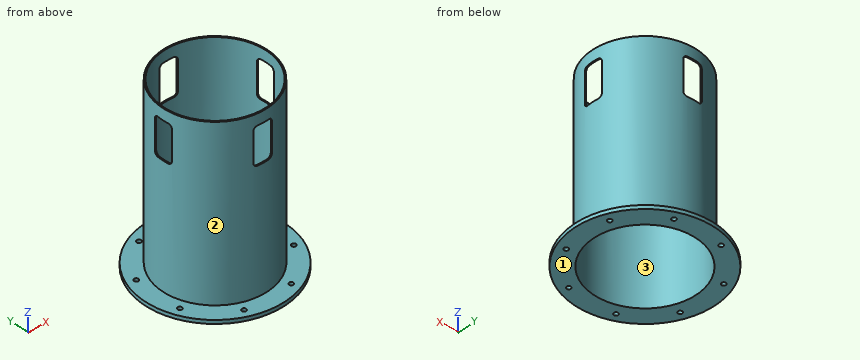
from build123d import *

# Parameters (mm, degrees)
SKETCH011_R      = 17.5
EXTRUDE005_DEPTH = 30
ARRAY004_COUNT   = 8
EXTRUDE_DEPTH    = 500
ARRAY_COUNT      = 4


with BuildPart() as extrude005:
    # Sketch011 (on Face4 of Cut) → Extrude005 (new body)
    with BuildSketch(Plane(origin=(0, 0, 2955), x_dir=(1, 0, 0), z_dir=(0, 0, -1))):
        with Locations((461.939766, 191.341716)):
            Circle(SKETCH011_R)
    extrude(amount=-EXTRUDE005_DEPTH)


with BuildPart() as array004:
    # Array004 base: copy of Extrude005
    add(extrude005.part)

    # Array004: Array004 ×8 about axis
    array004_axis = Axis((0, 0, 0), (0, 0, 1))


with BuildPart() as array004_1:
    add(array004.part)
    for i in range(1, ARRAY004_COUNT):
        add(array004.part.rotate(array004_axis, i * 360 / ARRAY004_COUNT))


with BuildPart() as array:
    # Sketch010 → Extrude (new body)
    with BuildSketch(Plane.XZ):
        with BuildLine():
            Line((-45, 3965), (45, 3965))
            ThreePointArc((45, 3965), (66.213203, 3973.786797), (75, 3995))
            Line((75, 3995), (75, 4235))
            ThreePointArc((75, 4235), (66.213203, 4256.213203), (45, 4265))
            Line((45, 4265), (-45, 4265))
            ThreePointArc((-45, 4265), (-66.213203, 4256.213203), (-75, 4235))
            Line((-75, 4235), (-75, 3995))
            ThreePointArc((-75, 3995), (-66.213203, 3973.786797), (-45, 3965))
        make_face()
    extrude(amount=EXTRUDE_DEPTH)

    # Array: Array ×4 about axis
    array_axis = Axis((0, 0, 0), (0, 0, 1))


with BuildPart() as array_1:
    add(array.part)
    for i in range(1, ARRAY_COUNT):
        add(array.part.rotate(array_axis, i * 360 / ARRAY_COUNT))


with BuildPart() as top001:
    # Sketch003 → Revolve003 (revolve)
    with BuildSketch(Plane.XZ):
        Polygon((569, 2985), (425, 2985), (425, 4355), (415, 4355), (415, 2955), (569, 2955), align=None)
    revolve(axis=Axis((0, 0, 0), (0, 0, 1)))

    # Cut: cut Array
    add(array_1.part, mode=Mode.SUBTRACT)

    # Cut004: cut Extrude005
    add(extrude005.part, mode=Mode.SUBTRACT)

    # Cut005: cut Array004
    add(array004_1.part, mode=Mode.SUBTRACT)


with BuildPart() as top001_1:
    # Cut005 placement: moved
    add(top001.part.moved(Location((0, 0, 50))))


solid = top001_1.part
Could you check a few things on this model? Use its own coordinates, in mm. Face numbers are marked on the shaded views. Give positions to 0.01 mm unless a question says otherwise; leave off trailing zeros. Order: outer loops, then holes, each group sorted by start corner. A loop starts at its lowest first (then second) coordinate and runs counter-clockwise, first axis right, second up. Notation, with made-up numbers: (-25.5, -35) - (-15.5, -35) arc R9 ccw to (-15.5, -19) - close; hole circle Ø3 at (16, 29). An arc over 180 degrees is marked (long way). One line per question, with ' | ' between items. Start each with the question number.
Item 1: I'm going to push flat-ended pins straight in: pin 1 Ø1.5 at (y, z) = (-345, 4107) entering from +X; pin 2 Ø10 at (y, z) = (-332.5, 3623.5) entering from -X; pin 3 Ø4 at (y, z) = (360, 4014) entering from +X; pin 4 Ø21 at (x, y) = (-461.94, 191.34) entering from +Z. Where does each tip first touch, or does it pass through?
Item 2: I want a section at C-C on z = 4162. Write out the boundary of the cut face in (x, y).
Item 3: I want a section at D-D on x = 263. Write out the boundary of the cut face in (y, z), then the cut area to 3 significant figures.
Item 4: I want a section at A-A on y = 0. Write out the boundary of the cut face in (x, z).
Item 5: Thinking about a two-plate mould opening in Y: for the marked faces 1, 2 and 3, which applies, pulls with the +Y half, pulls with the -Y half, needs draft (parallel to the pull), parting line crosses it, or undercut?
Item 6: I need wall thicknesses on probe 1 along Y at (x, z) = (-18, 3687.5); probe 2 along Z at (x, y) = (247, -447); probe 3 along Y at (x, z) = (369, 3530.5). Which ranges of each line are inside material? Lowest first, please. Write a range as [from, to].
Verdict:
1) pin 1: x = 249.23 | pin 2: x = -270.87 | pin 3: x = 229.04 | pin 4: through
2) outline: (-418.33, -75) arc R425 ccw to (-75, -418.33) - (-75, -408.17) arc R415 cw to (-408.17, -75) - close; (-418.33, 75) - (-408.17, 75) arc R415 cw to (-75, 408.17) - (-75, 418.33) arc R425 ccw to start; (75, -418.33) arc R425 ccw to (418.33, -75) - (408.17, -75) arc R415 cw to (75, -408.17) - close; (75, 408.17) arc R415 cw to (408.17, 75) - (418.33, 75) arc R425 ccw to (75, 418.33) - close
3) outline: (-504.57, 3005) - (-321.02, 3005) - (-321.02, 4405) - (-333.85, 4405) - (-333.85, 3035) - (-504.57, 3035) - close; (321.02, 3005) - (504.57, 3005) - (504.57, 3035) - (333.85, 3035) - (333.85, 4405) - (321.02, 4405) - close | area: 46,200 mm^2
4) outline: (-569, 3005) - (-415, 3005) - (-415, 4015) - (-425, 4015) - (-425, 3035) - (-569, 3035) - close; (-425, 4315) - (-415, 4315) - (-415, 4405) - (-425, 4405) - close; (415, 3005) - (569, 3005) - (569, 3035) - (425, 3035) - (425, 4015) - (415, 4015) - close; (415, 4315) - (425, 4315) - (425, 4405) - (415, 4405) - close
5) face 1: needs draft | face 2: parting line crosses it | face 3: undercut
6) probe 1: [-424.62, -414.61], [414.61, 424.62] | probe 2: [3005, 3035] | probe 3: [-210.86, -189.91], [189.91, 210.86]
